Here's how the part is built. I have some questions about the finished solid (model axes, mm). A direction names the side the tool comes from. Give positions to 0.01 mm unless a question says otherwise; leave off trailing zeros. Write each loop counter-clockwise with the first axis right and the second up, starting at its lowest first coordinate (ties: lowest second). Pieces come first, ordered by that corner, then holes. Notation, with made-up numbers: M 64.5,-34 L 68.5,-34 A18 cw 68.5,-15 Z; hole C 55.25,-2.75 d9. An arc over 180 degrees is marked long. Use one line per item in the form item = value. Start each with the question number.
from build123d import *

# Parameters (mm, degrees)
F0_R     = 6.985
F0_R_2   = 1.27
F1_DEPTH = 7.62
F2_R     = 4.445
F2_R_2   = 1.27
F3_DEPTH = 45.72
F5_DEPTH = 25.4
F6_DEPTH = 25.4
F7_R     = 2.54
F7_R_2   = 1.27
F8_DEPTH = 20.32
F9_DEPTH = 25.4


with BuildPart() as f1:
    # F0 (on Front) → F1 (new body)
    with BuildSketch(Plane.XZ):
        Circle(F0_R)
        Circle(F0_R_2, mode=Mode.SUBTRACT)
    extrude(amount=F1_DEPTH)

    # F2 (on face) → F3 (join)
    with BuildSketch(Plane.XZ.offset(7.62)):
        Circle(F2_R)
        Circle(F2_R_2, mode=Mode.SUBTRACT)
    extrude(amount=F3_DEPTH)

    # F4 (on Right) → F5 (cut)
    with BuildSketch(Plane.YZ):
        with BuildLine():
            ThreePointArc((-50.0528407257, 0.762), (-50.5916560929, 0.5388153673), (-50.8148407257, 0))
            Line((-50.8148407257, 0), (-50.0528407257, 0))
            Line((-50.0528407257, 0), (-50.0528407257, 0.762))
        make_face()
        with BuildLine():
            Line((-50.0528407257, 0), (-50.8148407257, 0))
            ThreePointArc((-50.8148407257, 0), (-50.5916560929, -0.5388153673), (-50.0528407257, -0.762))
            Line((-50.0528407257, -0.762), (-50.0528407257, 0))
        make_face()
        with BuildLine():
            Line((-50.0528407257, 0.762), (-50.0528407257, 0))
            Line((-50.0528407257, 0), (-49.2908407257, 0))
            ThreePointArc((-49.2908407257, 0), (-49.5140253584, 0.5388153673), (-50.0528407257, 0.762))
        make_face()
        with BuildLine():
            Line((-49.2908407257, 0), (-50.0528407257, 0))
            Line((-50.0528407257, 0), (-50.0528407257, -0.762))
            ThreePointArc((-50.0528407257, -0.762), (-49.5140253584, -0.5388153673), (-49.2908407257, 0))
        make_face()
        with BuildLine():
            Line((-34.8282884293, 0.7618434015), (-50.0528407257, 0.762))
            ThreePointArc((-50.0528407257, 0.762), (-49.5140253584, 0.5388153673), (-49.2908407257, 0))
            Line((-49.2908407257, 0), (-35.5748407257, 0))
            ThreePointArc((-35.5748407257, 0), (-35.3570902779, 0.533325815), (-34.8282884293, 0.7618434015))
        make_face()
        with BuildLine():
            ThreePointArc((-49.2908407257, 0), (-49.5140253584, -0.5388153673), (-50.0528407257, -0.762))
            Line((-50.0528407257, -0.762), (-34.8128407257, -0.762))
            ThreePointArc((-34.8128407257, -0.762), (-35.3516560929, -0.5388153673), (-35.5748407257, 0))
            Line((-35.5748407257, 0), (-49.2908407257, 0))
        make_face()
        with BuildLine():
            ThreePointArc((-34.0508407257, 0), (-34.2795149107, 0.5442495522), (-34.8282884293, 0.7618434015))
            ThreePointArc((-34.8282884293, 0.7618434015), (-35.3570902779, 0.533325815), (-35.5748407257, 0))
            Line((-35.5748407257, 0), (-34.0508407257, 0))
        make_face()
        with BuildLine():
            ThreePointArc((-35.5748407257, 0), (-35.3516560929, -0.5388153673), (-34.8128407257, -0.762))
            ThreePointArc((-34.8128407257, -0.762), (-34.2740253584, -0.5388153673), (-34.0508407257, 0))
            Line((-34.0508407257, 0), (-35.5748407257, 0))
        make_face()
    extrude(amount=-F5_DEPTH, mode=Mode.SUBTRACT)

    # F4 (on Right) → F6 (cut)
    with BuildSketch(Plane.YZ):
        with BuildLine():
            ThreePointArc((-50.0528407257, 0.762), (-50.5916560929, 0.5388153673), (-50.8148407257, 0))
            Line((-50.8148407257, 0), (-50.0528407257, 0))
            Line((-50.0528407257, 0), (-50.0528407257, 0.762))
        make_face()
        with BuildLine():
            Line((-50.0528407257, 0), (-50.8148407257, 0))
            ThreePointArc((-50.8148407257, 0), (-50.5916560929, -0.5388153673), (-50.0528407257, -0.762))
            Line((-50.0528407257, -0.762), (-50.0528407257, 0))
        make_face()
        with BuildLine():
            Line((-50.0528407257, 0.762), (-50.0528407257, 0))
            Line((-50.0528407257, 0), (-49.2908407257, 0))
            ThreePointArc((-49.2908407257, 0), (-49.5140253584, 0.5388153673), (-50.0528407257, 0.762))
        make_face()
        with BuildLine():
            Line((-49.2908407257, 0), (-50.0528407257, 0))
            Line((-50.0528407257, 0), (-50.0528407257, -0.762))
            ThreePointArc((-50.0528407257, -0.762), (-49.5140253584, -0.5388153673), (-49.2908407257, 0))
        make_face()
        with BuildLine():
            Line((-34.8282884293, 0.7618434015), (-50.0528407257, 0.762))
            ThreePointArc((-50.0528407257, 0.762), (-49.5140253584, 0.5388153673), (-49.2908407257, 0))
            Line((-49.2908407257, 0), (-35.5748407257, 0))
            ThreePointArc((-35.5748407257, 0), (-35.3570902779, 0.533325815), (-34.8282884293, 0.7618434015))
        make_face()
        with BuildLine():
            ThreePointArc((-49.2908407257, 0), (-49.5140253584, -0.5388153673), (-50.0528407257, -0.762))
            Line((-50.0528407257, -0.762), (-34.8128407257, -0.762))
            ThreePointArc((-34.8128407257, -0.762), (-35.3516560929, -0.5388153673), (-35.5748407257, 0))
            Line((-35.5748407257, 0), (-49.2908407257, 0))
        make_face()
        with BuildLine():
            ThreePointArc((-34.0508407257, 0), (-34.2795149107, 0.5442495522), (-34.8282884293, 0.7618434015))
            ThreePointArc((-34.8282884293, 0.7618434015), (-35.3570902779, 0.533325815), (-35.5748407257, 0))
            Line((-35.5748407257, 0), (-34.0508407257, 0))
        make_face()
        with BuildLine():
            ThreePointArc((-35.5748407257, 0), (-35.3516560929, -0.5388153673), (-34.8128407257, -0.762))
            ThreePointArc((-34.8128407257, -0.762), (-34.2740253584, -0.5388153673), (-34.0508407257, 0))
            Line((-34.0508407257, 0), (-35.5748407257, 0))
        make_face()
    extrude(amount=F6_DEPTH, mode=Mode.SUBTRACT)

    # F7 (on face) → F8 (cut)
    with BuildSketch(Plane.XZ.offset(53.34)):
        Circle(F7_R)
        Circle(F7_R_2, mode=Mode.SUBTRACT)
    extrude(amount=-F8_DEPTH, mode=Mode.SUBTRACT)

    # F9 (cut): a face of the model
    f9_faces = [f1.faces().sort_by_distance(p)[0] for p in [
        (-2.468157951, -33.02, 0),
    ]]
    extrude(f9_faces, amount=-F9_DEPTH, mode=Mode.SUBTRACT)


solid = f1.part
1) Suppose I cut it at A-A, the plane x = 0. List the corners of the cut face in (y, z) for me (3 decimals), and give its area (3 significant figures).
2) Thinking about a two-plate mould opening in Y: for faces 4 (the face through (-3, -43, -0.762)), 5 (the face through (1.5, 0, 0.1)), 6 (the face through (-0.17, -3.76, 1.26)), which applies, released by +Y, released by -Y, zero draft, split by the parting line, or undercut?
3) Will these pins go through, and if not, where does the flat tip stop? P1, Ø0.6, axis at x = -3.5, y = -40.5, coming from the -Z side; P2, Ø4, axis at y = -47.5, z = -3.5, coming from the +X side; P3, Ø4, axis at x = 0, z = 0, coming from the -Y side; P4, Ø1, axis at y = -41.5, z = -5, coming from the -X side.
4) Suppose I cut it at D-D, the plane z = -3. List the corners of the cut face in (x, y) for me.
5) Suppose I cut it at C-C, the plane x = -3. List the corners of the cut face in (y, z) for me.
6) Please list where these lines run through material, in increasing order: line 1 (Z direction, x = 0, y = -1.5) (3 decimals); line 2 (Z direction, x = 0, y = -29.5) (3 decimals); line 3 (Y direction, x = -4.25, z = -2.5).
7) Suppose I cut it at B-B, the plane y = -38.5. List the corners of the cut face in (x, z) for me (3 decimals).
8) On a 3-axis mill with a long thin cutter (end or side, diameter ignored), from which of +Z, -Z, +X, -X, +Y, -Y can I reach the whole of each face in a straight line? I mean faces 1 (the face through (2, -53.34, -2)), 2 (the face through (1.1, -7.62, -1.1)), 3 (the face through (3, -43, -0.762)). Say none if no direction works.
Checks:
q1.outline = M -53.34,-4.445 L -7.62,-4.445 L -7.62,-6.985 L 0,-6.985 L 0,-1.27 L -7.62,-1.27 L -7.62,-2.54 L -53.34,-2.54 Z; M -53.34,2.54 L -7.62,2.54 L -7.62,1.27 L 0,1.27 L 0,6.985 L -7.62,6.985 L -7.62,4.445 L -53.34,4.445 Z
q1.area = 261 mm^2
q2.face_4 = undercut
q2.face_5 = released by +Y
q2.face_6 = zero draft
q3.P1 = -3.09
q3.P2 = 4.18
q3.P3 = -7.62
q3.P4 = through
q4.outline = M -6.31,-7.62 L -3.28,-7.62 L -3.28,-53.34 L 3.28,-53.34 L 3.28,-7.62 L 6.31,-7.62 L 6.31,0 L -6.31,0 Z
q5.outline = M -53.34,-3.28 L -7.62,-3.28 L -7.62,-6.31 L 0,-6.31 L 0,6.31 L -7.62,6.31 L -7.62,3.28 L -53.34,3.28 Z; hole M -50.05,-0.76 L -34.81,-0.76 A0.76 ccw long -34.83,0.76 L -50.05,0.76 A0.76 ccw Z
q6.line_1 = -6.985 to -1.27, 1.27 to 6.985
q6.line_2 = -4.445 to -2.54, 2.54 to 4.445
q6.line_3 = -7.62 to 0
q7.outline = M -4.379,-0.762 A4.445 ccw 4.379,-0.762 L 2.423,-0.762 A2.54 cw -2.423,-0.762 Z; M -4.379,0.762 L -2.423,0.762 A2.54 cw 2.423,0.762 L 4.379,0.762 A4.445 ccw Z
q8.face_1 = +Z, -Z, +X, -X, -Y
q8.face_2 = -Y
q8.face_3 = +X, -X
